Design review of the part built by this model. Coordinates are the model's own, in mm. Face numbers are marked on the shaded views. Give positions to 0.01 mm unless a question says otherwise; leave off trailing zeros. Order: outer loops, then holes, each group sorted by start corner. A loop starts at its lowest first (then second) coordinate and runs counter-clockwise, first axis right, second up.
```python
from build123d import *

# Parameters (mm, degrees)
SKETCH1_R           = 41.275
SKETCH1_R_2         = 3.175
BOSS_EXTRUDE1_DEPTH = 5.842
SKETCH7_R           = 41.275
SKETCH7_R_2         = 39.487499946
CUT_EXTRUDE3_DEPTH  = 59.663278241
SKETCH8_W           = 5.842
SKETCH8_H           = 12.7
SKETCH8_W_2         = 12.7
SKETCH8_H_2         = 5.842
CUT_EXTRUDE4_DEPTH  = 57.148501921
SKETCH9_R           = 41.275
SKETCH9_R_2         = 39.487499946
BOSS_EXTRUDE2_DEPTH = 5.842


with BuildPart() as part:
    # Sketch1 → Boss-Extrude1 (new body)
    with BuildSketch(Plane.XY):
        Circle(SKETCH1_R)
        with Locations((0, 34.925)):
            Circle(SKETCH1_R_2, mode=Mode.SUBTRACT)
        with Locations((30.245937227, -17.4625)):
            Circle(SKETCH1_R_2, mode=Mode.SUBTRACT)
        with Locations((-30.245937227, -17.4625)):
            Circle(SKETCH1_R_2, mode=Mode.SUBTRACT)
        with BuildLine():
            Line((-25.3015625, -12.8), (25.3015625, -12.8))
            ThreePointArc((25.3015625, -12.8), (25.640316502, -12.940316502), (25.5, -12.6015625))
            Line((25.5, -12.6015625), (25.5, 12.6015625))
            ThreePointArc((25.5, 12.6015625), (25.640316502, 12.940316502), (25.3015625, 12.8))
            Line((25.3015625, 12.8), (-25.3015625, 12.8))
            ThreePointArc((-25.3015625, 12.8), (-25.640316502, 12.940316502), (-25.5, 12.6015625))
            Line((-25.5, 12.6015625), (-25.5, -12.6015625))
            ThreePointArc((-25.5, -12.6015625), (-25.640316502, -12.940316502), (-25.3015625, -12.8))
        make_face(mode=Mode.SUBTRACT)
    extrude(amount=BOSS_EXTRUDE1_DEPTH)

    # Sketch7 → Cut-Extrude3 (cut, through all)
    with BuildSketch(Plane(origin=(0, 0, 0), x_dir=(-1, 0, 0), z_dir=(0, 0, -1))):
        Circle(SKETCH7_R)
        Circle(SKETCH7_R_2, mode=Mode.SUBTRACT)
    extrude(amount=-CUT_EXTRUDE3_DEPTH, mode=Mode.SUBTRACT)

    # Sketch8 → Cut-Extrude4 (cut, through all)
    with BuildSketch(Plane(origin=(0, 0, 0), x_dir=(-1, 0, 0), z_dir=(0, 0, -1))):
        with Locations((-28.421, 0)):
            Rectangle(SKETCH8_W, SKETCH8_H)
        with Locations((-12.599996942, 15.721)):
            Rectangle(SKETCH8_W_2, SKETCH8_H_2)
        with Locations((12.800003058, 15.721)):
            Rectangle(SKETCH8_W_2, SKETCH8_H_2)
        with Locations((12.800003058, -15.721)):
            Rectangle(SKETCH8_W_2, SKETCH8_H_2)
        with Locations((-12.599996942, -15.721)):
            Rectangle(SKETCH8_W_2, SKETCH8_H_2)
        with Locations((28.421, 0)):
            Rectangle(SKETCH8_W, SKETCH8_H)
    extrude(amount=-CUT_EXTRUDE4_DEPTH, mode=Mode.SUBTRACT)

    # Sketch9 → Boss-Extrude2 (add)
    with BuildSketch(Plane(origin=(0, 0, 0), x_dir=(-1, 0, 0), z_dir=(0, 0, -1))):
        Circle(SKETCH9_R)
        Circle(SKETCH9_R_2, mode=Mode.SUBTRACT)
    extrude(amount=-BOSS_EXTRUDE2_DEPTH)


solid = part.part
```
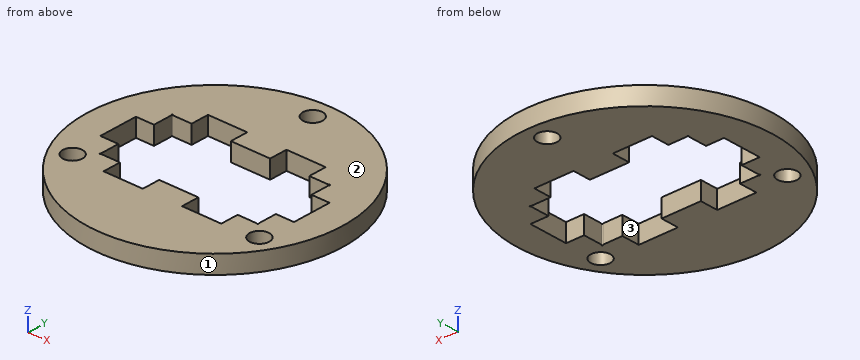
1. For pin 1 (1.5 mm diameter, centred on y = 3, z = 1, fed in from +X); pin 2 (1 mm diameter, centred on x = 21, z = 2.5, fed in from -Y); pin 3 (1.8 mm diameter, centred on y = 15.5, z = 2.5, fed in from +X), all flat-tipped, find the tip position at first contact; note any pin that passes through.
Recorded:
pin 1: stops at x = 41.21
pin 2: stops at y = -35.82
pin 3: stops at x = 38.61
2. For line 1 along Y through (x, z) = (0, 2.05) (3 decimals); line 2 along Y through (x, z) = (28, 0.35); line 3 along X through (y, z) = (-19, 4.2), list the stretches that pass through material, from the lowest coordinate up.
Recorded:
line 1: y = -41.275 to -12.8, 12.8 to 31.75, 38.1 to 41.275
line 2: y = -30.33 to -19.71, -15.22 to -6.35, 6.35 to 30.33
line 3: x = -36.64 to -33.02, -27.47 to 27.47, 33.02 to 36.64
3. Take a section at A-A (x = 0). State the section outline as (y, z) points (3 decimals).
Recorded:
outline: (-41.275, 0) - (-12.8, 0) - (-12.8, 5.842) - (-41.275, 5.842) - close; (12.8, 0) - (31.75, 0) - (31.75, 5.842) - (12.8, 5.842) - close; (38.1, 0) - (41.275, 0) - (41.275, 5.842) - (38.1, 5.842) - close
4. Take a section at B-B (y = 0). State the section outline as (x, z) points (3 decimals), then the cut area to 3 significant figures.
Recorded:
outline: (-41.275, 0) - (-31.342, 0) - (-31.342, 5.842) - (-41.275, 5.842) - close; (31.342, 0) - (41.275, 0) - (41.275, 5.842) - (31.342, 5.842) - close
area: 116 mm2
5. Take a section at D-D (z = 1.3). State how many separate pieces and enclosed holes the cut face has, then the cut area to 3 significant figures.
Recorded:
separate pieces: 1
enclosed holes: 4
area: 3,510 mm2
6. Take a section at C-C (x = 17.5). State the section outline as (y, z) points.
Recorded:
outline: (-37.38, 0) - (-18.64, 0) - (-18.64, 5.84) - (-37.38, 5.84) - close; (18.64, 0) - (37.38, 0) - (37.38, 5.84) - (18.64, 5.84) - close
7. Draft analysis for pull direction Y (two halves, no side actions). For the marked faces 1, 2 and 3, state which applies: pulls with the +Y half, pulls with the -Y half, needs draft (parallel to the pull), parting line crosses it, or undercut.
Recorded:
face 1: parting line crosses it
face 2: needs draft
face 3: undercut
